Job drawing, mm, ordinate dimensions from the low corner. One solid piece. A direction names the side the tool comes from. Give positions to 0.01 mm unless a question says otherwise; leave off trailing zeros. Order: outer loops, then holes, each group sorted by start corner. A loop starts at its lowest first (then second) coordinate and runs counter-clockwise, first axis right, second up.
Item 1: Wall check: L1, parallel to X at y = 5, z = 12 (1 decimal); L2, parallel to Z at x = 33, y = 10.5; L3, parallel to Y at x = 3.5, z = 13 (1 decimal). Give the ranges that are in metal, low to high.
Item 2: Which spindle directions (+Z, -Z, +X, -X, +Y, -Y) get a long thin tool onto all of the face, cutting with end or side? Do the marked faces 1, 2 and 3. Say none if no direction does.
Item 3: Band-saw the part on A-A on x = 25. Count the separate pieces of the cut face and the enclosed holes in it, plus the area to 3 significant figures.
Item 4: Band-saw the part on B-B on z = 19. Give the cut face in (x, y) (1 decimal).
Item 5: Band-saw the part on D-D on y = 13.5. Give the cut face in (x, z).
Item 6: Two-plate mould, pull along Z, no slides. Class the marked faces 4, 5 and 6: released by +Z, released by -Z, zero draft, split by the parting line, or undercut.
Item 7: Flat gauge pins, fed straight in: P1, Ø8, axis at x = 33.5, z = 20, coming from the +Y side (1 decimal); P2, Ø12, axis at y = 31.5, z = 5.5, coming from the -X side (1 decimal); P3, Ø10, axis at y = 30.5, z = 20, coming from the -X side; P4, Ø5, axis at x = 9, z = 15.5, coming from the +Y side (1 decimal). Where does each tip first touch, or does it go through?
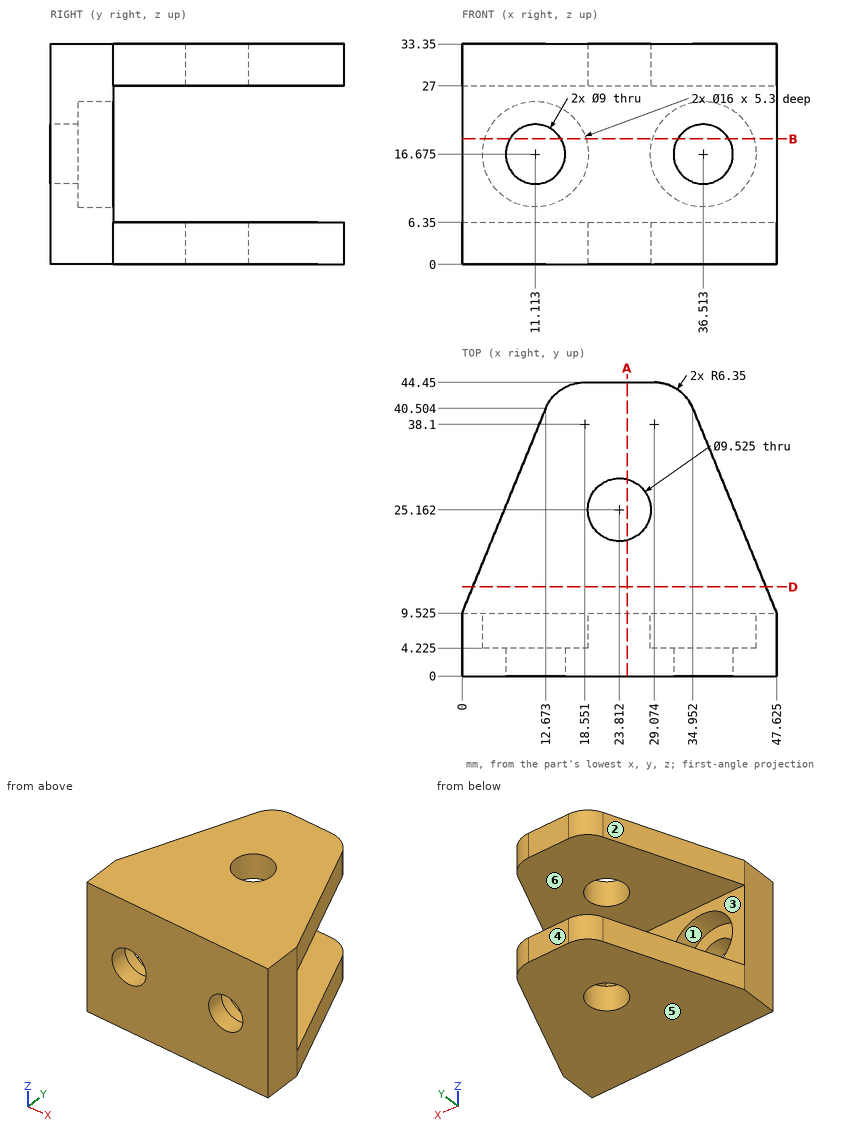
The answers:
1. L1: x = 0 to 4.6, 17.6 to 30, 43 to 47.6
1. L2: z = 0 to 6.35, 27 to 33.35
1. L3: y = 0 to 9.5
2. face 1: +Y
2. face 2: +Z, -Z, -X, +Y
2. face 3: +X, -X, +Y
3. separate pieces: 3
3. enclosed holes: 0
3. area: 644 mm2
4. outline: (0, 0) - (7.3, 0) - (7.3, 4.2) - (3.5, 4.2) - (3.5, 9.5) - (0, 9.5) - close; (15, 0) - (32.7, 0) - (32.7, 4.2) - (28.9, 4.2) - (28.9, 9.5) - (18.8, 9.5) - (18.8, 4.2) - (15, 4.2) - close; (40.4, 0) - (47.6, 0) - (47.6, 9.5) - (44.2, 9.5) - (44.2, 4.2) - (40.4, 4.2) - close
5. outline: (1.63, 0) - (46, 0) - (46, 6.35) - (1.63, 6.35) - close; (1.63, 27) - (46, 27) - (46, 33.35) - (1.63, 33.35) - close
6. face 4: zero draft
6. face 5: released by -Z
6. face 6: undercut
7. P1: stops at y = 9.5
7. P2: stops at x = 6.5
7. P3: passes through
7. P4: stops at y = 4.2
